Source: three-view drawing plus pictorial views. Frame: mm from the lowest corner of the part. A direction names the side the tool comes from. Give positions to 0.01 mm unless a question says otherwise; leave off trailing zeros. Write each loop counter-clockwise with the first axis right and the second up, starting at its lowest first coordinate (ties: lowest second). Pieces come first, ordered by that corner, then holes. Notation, with made-up numbers: (-12, 5.5) -> (-5, 5.5) arc R32 ccw to (-5, 36.5) -> close; hole circle Ø5 at (74, 19). An arc over 180 degrees is marked (long way). Write item = value, one per line.
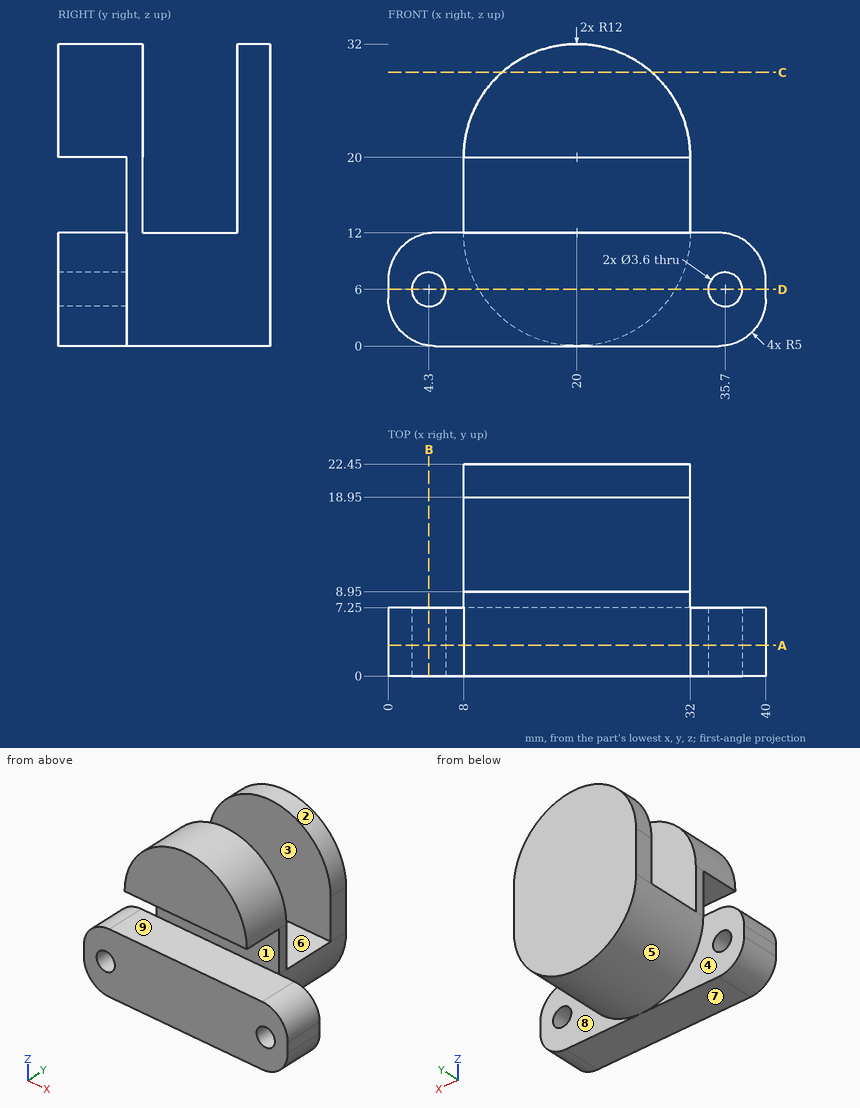
1) Cut plane D-D (z = 6). Return the cut outline in (x, y).
Computed:
outline = (0, 0) -> (2.5, 0) -> (2.5, 7.25) -> (0, 7.25) -> close; (6.1, 0) -> (33.9, 0) -> (33.9, 7.25) -> (30.39, 7.25) -> (30.39, 22.45) -> (9.61, 22.45) -> (9.61, 7.25) -> (6.1, 7.25) -> close; (37.5, 0) -> (40, 0) -> (40, 7.25) -> (37.5, 7.25) -> close
2) Material intervals for L1, parallel to Y at x = 20, z = 22; L2, parallel to Y at x = 32, z = 10; L3, parallel to Y at x = 29, z = 14, sorted ascending.
Computed:
L1 = 0 to 8.95, 18.95 to 22.45
L2 = 0 to 7.25
L3 = 7.25 to 8.95, 18.95 to 22.45
3) Contact query for flat-ended pins moving along their axis: pin 1 (1.5 mm diameter, centred on x = 11, y = 5, fed in from +Z); pin 2 (8 mm diameter, centred on y = 6, z = 19.5, fed in from -X); pin 3 (0.8 mm diameter, centred on y = 8, z = 14.5, fed in from +X); pin 4 (3 mm diameter, centred on x = 35.5, y = 9, fed in from -Z). Output: stop coordinate, or through.
Computed:
pin_1 = 28.71
pin_2 = 8
pin_3 = 32
pin_4 = through
4) Draft query along Y for the marked faces 1, 2, 3 and 4. Return one class per face: pulls with the +Y half, pulls with the -Y half, needs draft (parallel to the pull), parting line crosses it, or undercut.
Computed:
face_1 = pulls with the -Y half
face_2 = needs draft
face_3 = undercut
face_4 = pulls with the +Y half
5) Access query for the marked faces 5, 6, 7, 8 and 9. Directions: +Z, -Z, +X, -X, +Y, -Y. A direction counts if a zero-diameter tool reaches every point of the face in a straight line with its end or side. Return the directions, or none.
Computed:
face_5 = -Z, +Y
face_6 = +Z, +X, -X
face_7 = -Z, +X, -X, +Y, -Y
face_8 = -Z, +X, +Y
face_9 = +X, -X, -Y
6) Cut plane A-A (y = 3.25). Return the cut outline in (x, z).
Computed:
outline = (0, 5) arc R5 ccw to (5, 0) -> (35, 0) arc R5 ccw to (40, 5) -> (40, 7) arc R5 ccw to (35, 12) -> (5, 12) arc R5 ccw to (0, 7) -> close; (8, 20) -> (32, 20) arc R12 ccw to start; hole circle Ø3.6 at (4.3, 6); hole circle Ø3.6 at (35.7, 6)
7) Cut plane B-B (x = 4.3). Return the cut outline in (y, z), then the cut area to 3 significant figures.
Computed:
outline = (0, 0.05) -> (7.25, 0.05) -> (7.25, 4.2) -> (0, 4.2) -> close; (0, 7.8) -> (7.25, 7.8) -> (7.25, 11.95) -> (0, 11.95) -> close
area = 60.2 mm²
8) Cut plane C-C (z = 29). Return the cut outline in (x, y), then the cut area to 3 significant figures.
Computed:
outline = (12.06, 0) -> (27.94, 0) -> (27.94, 8.95) -> (12.06, 8.95) -> close; (12.06, 18.95) -> (27.94, 18.95) -> (27.94, 22.45) -> (12.06, 22.45) -> close
area = 198 mm²
